from build123d import *

# Parameters (mm, degrees)
F0_R     = 2.5
F1_DEPTH = 12
F2_R     = 8
F2_R_2   = 2.5
F3_DEPTH = 2
F4_R     = 3
F5_DEPTH = 36


with BuildPart() as f1:
    # F0 (on Top) → F1 (new body)
    with BuildSketch(Plane.XY):
        Circle(F0_R)
    extrude(amount=F1_DEPTH)

    # F2 (on face) → F3 (join)
    with BuildSketch(Plane.XY.offset(12)):
        Circle(F2_R)
        Circle(F2_R_2, mode=Mode.SUBTRACT)
        Circle(F2_R)
    extrude(amount=F3_DEPTH)

    # F4 (on face) → F5 (join)
    with BuildSketch(Plane.XY.offset(14)):
        Circle(F4_R)
    extrude(amount=F5_DEPTH)


solid = f1.part
The model under review builds one solid part; all positions refer to its coordinate system, in mm. A direction names the side the tool comes from. Coordinates: 2 decimals unless noted, no trailing zeros. Loops run counter-clockwise (first coordinate to the right, second up) from the corner with the lowest first, then second, coordinate; pieces in that order, holes last. Notation, with made-up numbers: (15, 31) -> (61, 31) arc R18 cw to (61, 44) -> close; hole circle Ø3 at (25.5, -40). An arc over 180 degrees is marked (long way). Use a Markdown table: item, result. Add a question column.
1. Add section A-A on x = 0. Write out the cut boundary in (y, z), plus the area to 3 significant figures.
2. Clearance check with flat-ended pins moving along their axes: pin 1 Ø3 at (x, y) = (-4, -3) entering from -Z; pin 2 Ø8 at (y, z) = (5.5, 22.5) entering from -X; pin 3 Ø6 at (x, z) = (5, 8.5) entering from +Y. State where each tip first meets the part, or that it passes through.
3. Add section C-C on z = 7. Write out the cut boundary in (x, y).
4. To check wall thickness, follow line 1 (Z direction, x = -1, y = 3.75); line 2 (Y direction, x = 2.25, z = 16); line 3 (X direction, y = -2, z = 10.5). State the ranges of each line that lie inside material, in increasing order.
5. Machinability: for faces 1 (the face through (0, 0, 0)), 2 (the face through (-3, 0, 32)), 3 (the face through (-0.54, -2.44, 5.92)), which of the approach directions +Z, -Z, +X, -X, +Y, -Y give a long, thin tool a straight path to every point of the face, cutting with its end or side? Answer none if there is none.
6. Add section D-D on y = -6.75. Write out the cut boundary in (x, z).
Returned:
| question | item | result |
|---|---|---|
| 1 | outline | (-8, 12) -> (-2.5, 12) -> (-2.5, 0) -> (2.5, 0) -> (2.5, 12) -> (8, 12) -> (8, 14) -> (3, 14) -> (3, 50) -> (-3, 50) -> (-3, 14) -> (-8, 14) -> close |
| 1 | area | 308 mm² |
| 2 | pin 1 | stops at z = 12 |
| 2 | pin 2 | stops at x = -2.6 |
| 2 | pin 3 | stops at y = 1.5 |
| 3 | outline | circle Ø5 at (0, 0) |
| 4 | line 1 | z = 12 to 14 |
| 4 | line 2 | y = -1.98 to 1.98 |
| 4 | line 3 | x = -1.5 to 1.5 |
| 5 | face 1 | -Z, +X, -X, +Y, -Y |
| 5 | face 2 | +Z |
| 5 | face 3 | -Z |
| 6 | outline | (-4.29, 12) -> (4.29, 12) -> (4.29, 14) -> (-4.29, 14) -> close |
